The listing builds one solid part. Answer for the finished solid, in the listing's coordinates (mm). Coordinates: 2 decimals unless noted, no trailing zeros. Order: outer loops, then holes, each group sorted by start corner. A loop starts at its lowest first (then second) coordinate and runs counter-clockwise, first axis right, second up. Notation, with made-up numbers: (15, 39) - (51, 39) arc R19 cw to (51, 49) - close; hole circle Ø1 at (51.5, -22.75). An arc over 180 degrees is marked (long way). One line per item, written item: value. Start each with the question number.
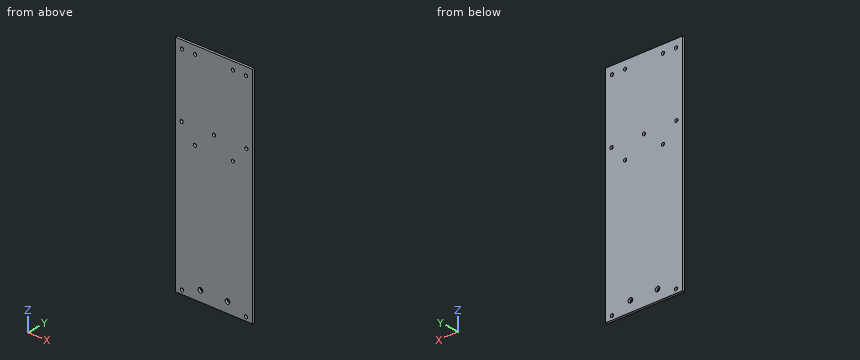
```python
from build123d import *

# Parameters (mm, degrees)
SKETCH1_W           = 100
SKETCH1_H           = 120
SKETCH1_R           = 2.1
BOSS_EXTRUDE1_DEPTH = 3
SKETCH2_R           = 2.1
CUT_EXTRUDE1_DEPTH  = 10
SKETCH3_W           = 100
SKETCH3_H           = 3
BOSS_EXTRUDE2_DEPTH = 160
SKETCH4_R           = 3
SKETCH4_R_2         = 2.1
CUT_EXTRUDE2_DEPTH  = 160


with BuildPart() as part:
    # Sketch1 → Boss-Extrude1 (new body)
    with BuildSketch(Plane(origin=(0, 0, 0), x_dir=(1, 0, 0), z_dir=(0, 1, 0))):
        Rectangle(SKETCH1_W, SKETCH1_H)
        with Locations(Location((41.5, -50, 0), (0, 0, 90))):
            Circle(SKETCH1_R, mode=Mode.SUBTRACT)
        with Locations(Location((-41.5, -50, 0), (0, 0, 270))):
            Circle(SKETCH1_R, mode=Mode.SUBTRACT)
        with Locations(Location((-42, 30, 0), (0, 0, 270))):
            Circle(SKETCH1_R, mode=Mode.SUBTRACT)
        with Locations(Location((0, 30, 0), (0, 0, 270))):
            Circle(SKETCH1_R, mode=Mode.SUBTRACT)
        with Locations(Location((42, 30, 0), (0, 0, 270))):
            Circle(SKETCH1_R, mode=Mode.SUBTRACT)
    extrude(amount=BOSS_EXTRUDE1_DEPTH)

    # Sketch2 → Cut-Extrude1 (cut)
    with BuildSketch(Plane.XZ):
        with Locations(Location((-24.5, -50, 0), (0, 0, 270))):
            Circle(SKETCH2_R)
        with Locations(Location((24.5, -50, 0), (0, 0, 270))):
            Circle(SKETCH2_R)
        with Locations(Location((24.5, 50, 0), (0, 0, 270))):
            Circle(SKETCH2_R)
        with Locations(Location((-24.5, 50, 0), (0, 0, 270))):
            Circle(SKETCH2_R)
    extrude(amount=-CUT_EXTRUDE1_DEPTH, mode=Mode.SUBTRACT)

    # Sketch3 → Boss-Extrude2 (add)
    with BuildSketch(Plane(origin=(0, 0, -60), x_dir=(-1, 0, 0), z_dir=(0, 0, -1))):
        with Locations((0, 1.5)):
            Rectangle(SKETCH3_W, SKETCH3_H)
    extrude(amount=BOSS_EXTRUDE2_DEPTH)

    # Sketch4 → Cut-Extrude2 (cut)
    with BuildSketch(Plane.XZ):
        with Locations(Location((17.5, -206.7, 0), (0, 0, 270))):
            Circle(SKETCH4_R)
        with Locations(Location((-17.5, -206.7, 0), (0, 0, 270))):
            Circle(SKETCH4_R)
        with Locations(Location((-41.5, -215, 0), (0, 0, 270))):
            Circle(SKETCH4_R_2)
        with Locations(Location((41.5, -215, 0), (0, 0, 270))):
            Circle(SKETCH4_R_2)
    extrude(amount=-CUT_EXTRUDE2_DEPTH, mode=Mode.SUBTRACT)


solid = part.part
```
(1) The part is cut by section B-B on x = -17.5. Determine the outline of the cut face in (y, z).
(2) Consider probe 1 along X at (y, z) = (2.5, -207); probe 2 along X at (y, z) = (2.05, 50); probe 3 along X at (y, z) = (1.95, -30). Determine where each line is inside the solid, lowest interval first.
(3) The part is cut by section A-A on z = -206.7. Determine the outline of the cut face in (x, y), plus the area to 3 significant figures.
Completed:
1. outline: (0, -220) - (3, -220) - (3, -209.7) - (0, -209.7) - close; (0, -203.7) - (3, -203.7) - (3, 60) - (0, 60) - close
2. probe 1: x = -50 to -20.48, -14.52 to 14.52, 20.48 to 50
2. probe 2: x = -50 to -43.6, -39.4 to -26.6, -22.4 to 22.4, 26.6 to 39.4, 43.6 to 50
2. probe 3: x = -50 to -44.1, -39.9 to -2.1, 2.1 to 39.9, 44.1 to 50
3. outline: (-50, 0) - (-20.5, 0) - (-20.5, 3) - (-50, 3) - close; (-14.5, 0) - (14.5, 0) - (14.5, 3) - (-14.5, 3) - close; (20.5, 0) - (50, 0) - (50, 3) - (20.5, 3) - close
3. area: 264 mm2
